from build123d import *

# Parameters (mm, degrees)
SKETCH1_W           = 88.9
SKETCH1_H           = 30.48
BOSS_EXTRUDE1_DEPTH = 3.175
BOSS_EXTRUDE2_DEPTH = 10.16
SKETCH3_W           = 68.58
SKETCH3_H           = 20.32
SKETCH3_W_2         = 10.16
CUT_EXTRUDE1_DEPTH  = 95.751277696
SKETCH5_R           = 2.8448
CUT_EXTRUDE2_DEPTH  = 12.7
CUT_EXTRUDE3_DEPTH  = 95.399536545
FILLET1_R           = 2.54


# Read off the part's stored shape, not the designer's step: Mirror4
with BuildPart() as part:
    # Sketch1 → Boss-Extrude1 (new body)
    with BuildSketch(Plane(origin=(0, 0, 0), x_dir=(1, 0, 0), z_dir=(0, 1, 0))):
        with Locations((-44.45, -15.24)):
            Rectangle(SKETCH1_W, SKETCH1_H)
    extrude(amount=BOSS_EXTRUDE1_DEPTH)

    # Sketch2 → Boss-Extrude2 (add)
    with BuildSketch(Plane.XY.offset(30.48)):
        with BuildLine():
            Line((-68.58, 3.175), (-65.151, 12.065))
            Line((-65.151, 12.065), (-54.991, 12.065))
            ThreePointArc((-54.991, 12.065), (-46.99, 4.064), (-38.989, 12.065))
            Line((-38.989, 12.065), (-28.829, 12.065))
            Line((-28.829, 12.065), (-25.4, 3.175))
            Line((-25.4, 3.175), (-68.58, 3.175))
        make_face()
    extrude(amount=-BOSS_EXTRUDE2_DEPTH)

    # Sketch3 → Cut-Extrude1 (cut, through all)
    with BuildSketch(Plane(origin=(0, 0, 0), x_dir=(1, 0, 0), z_dir=(0, 1, 0))):
        with Locations((-54.61, -10.16)):
            Rectangle(SKETCH3_W, SKETCH3_H)
        with Locations((-5.08, -10.16)):
            Rectangle(SKETCH3_W_2, SKETCH3_H)
    extrude(amount=CUT_EXTRUDE1_DEPTH, mode=Mode.SUBTRACT)

    # Sketch5 → Cut-Extrude2 (cut)
    with BuildSketch(Plane(origin=(0, 12.065, 0), x_dir=(1, 0, 0), z_dir=(0, 1, 0))):
        with Locations(Location((-33.909, -25.4, 0), (0, 0, 180))):
            Circle(SKETCH5_R)
        with Locations(Location((-60.071, -25.4, 0), (0, 0, 180))):
            Circle(SKETCH5_R)
    extrude(amount=-CUT_EXTRUDE2_DEPTH, mode=Mode.SUBTRACT)

    # Sketch6 → Cut-Extrude3 (cut, through all)
    with BuildSketch(Plane(origin=(0, 3.175, 0), x_dir=(1, 0, 0), z_dir=(0, 1, 0))):
        with BuildLine():
            Line((-81.28, -23.0505), (-73.66, -23.0505))
            ThreePointArc((-73.66, -23.0505), (-71.3105, -25.4), (-73.66, -27.7495))
            Line((-73.66, -27.7495), (-81.28, -27.7495))
            ThreePointArc((-81.28, -27.7495), (-83.6295, -25.4), (-81.28, -23.0505))
        make_face()
        with BuildLine():
            Line((-17.78, -23.0505), (-10.16, -23.0505))
            ThreePointArc((-10.16, -23.0505), (-7.8105, -25.4), (-10.16, -27.7495))
            Line((-10.16, -27.7495), (-17.78, -27.7495))
            ThreePointArc((-17.78, -27.7495), (-20.1295, -25.4), (-17.78, -23.0505))
        make_face()
    extrude(amount=-CUT_EXTRUDE3_DEPTH, mode=Mode.SUBTRACT)

    # Mirror4: part across plane


with BuildPart() as part_1:
    add(part.part)
    add(part.part.mirror(Plane.XY))

    # Fillet1
    fillet1_edges = [part_1.edges().sort_by_distance(p)[0] for p in [
        (0, 3.175, 25.4),
        (-88.9, 1.5875, -30.48),
        (0, 3.175, -25.4),
        (-78.74, 3.175, -30.48),
        (0, 1.5875, -30.48),
        (-12.7, 3.175, -30.48),
        (-68.58, 3.175, -25.4),
        (-27.1145, 7.62, -30.48),
        (-25.4, 3.175, -25.4),
        (-66.8655, 7.62, -30.48),
        (-27.1145, 7.62, -20.32),
        (-66.8655, 7.62, -20.32),
        (-12.7, 3.175, 30.48),
        (-88.9, 3.175, -25.4),
        (-22.86, 3.175, -20.32),
        (-78.74, 3.175, -20.32),
        (-88.9, 1.5875, -20.32),
        (-20.32, 1.5875, -20.32),
        (-25.4, 3.175, 25.4),
        (-66.8655, 7.62, 20.32),
        (0, 1.5875, -20.32),
        (-68.58, 3.175, 25.4),
        (-5.08, 3.175, -20.32),
        (-10.16, 1.5875, -20.32),
        (-27.1145, 7.62, 20.32),
        (-27.1145, 7.62, 30.48),
        (-66.8655, 7.62, 30.48),
        (-88.9, 3.175, 25.4),
        (-22.86, 3.175, 20.32),
        (-78.74, 3.175, 20.32),
        (-88.9, 1.5875, 20.32),
        (-20.32, 3.175, 0),
        (-20.32, 1.5875, 20.32),
        (0, 1.5875, 20.32),
        (-10.16, 3.175, 0),
        (-5.08, 3.175, 20.32),
        (-10.16, 1.5875, 20.32),
        (-78.74, 3.175, 30.48),
        (0, 1.5875, 30.48),
        (-88.9, 1.5875, 30.48),
    ]]
    fillet(fillet1_edges, radius=FILLET1_R)


solid = part_1.part
CAD build for the part. Positions are in the model's coordinates, mm. A direction names the side the tool comes from. Round coordinates to 2 decimals unless told otherwise and drop trailing zeros. Write each loop counter-clockwise with the first axis right and the second up, starting at its lowest first coordinate (ties: lowest second). Pieces come first, ordered by that corner, then holes. Notation, with made-up numbers: (-24.75, 12.25) -> (21.25, 12.25) arc R20 ccw to (21.25, 40.25) -> close; hole circle Ø9 at (-11.5, -4). An arc over 180 degrees is marked (long way). Answer as a JSON object with one key per item and string values.
(1) Band-saw the part on A-A, the plane z = 25.4. Count the separate pieces of the cut face and the enclosed holes in it, then the cut area to 3 significant figures.
Reported:
{"separate pieces": "5", "enclosed holes": "0", "area": "318 mm^2"}
(2) Which spindle directions (+Z, -Z, +X, -X, +Y, -Y) get a long thin tool onto all of the face, cutting with end or side? Do faces 4 (the face through (-5.116, 2.411, 21.044)), 5 (the face through (-78.454, 2.451, -21.084)), 6 (the face through (-48, 3, -20.32)). Say none if no direction does.
Reported:
{"face 4": "+X, +Y", "face 5": "-X, +Y", "face 6": "-X, +Y, -Y"}
(3) Band-saw the part on B-B, the plane x = -50.5. List the corners of the cut face in (y, z).
Reported:
{"outline": "(0, -30.48) -> (4.88, -30.48) -> (4.88, -20.32) -> (0, -20.32) -> close; (0, 20.32) -> (4.88, 20.32) -> (4.88, 30.48) -> (0, 30.48) -> close"}
(4) Two-plate mould, pull along X, no slides. Class faces 1 (the face through (-88.176, 2.411, -25.364)), 2 (the face through (-25.08, 3.61, -25.36)), 3 (the face through (-20.13, 1.61, 25.45)): +X half, -X half, draft (parallel to the pull), parting line (faces both ways), or undercut.
Reported:
{"face 1": "-X half", "face 2": "+X half", "face 3": "undercut"}
(5) Pin check, flat tips, straight feed: P1, Ø3, axis at y = 2.5, z = 3, coming from the +X side; P2, Ø4, axis at x = -45, z = 23.5, coming from the +Y side; P3, Ø1, axis at x = -16, y = 1.5, coming from the -Z side. Stop position of each tip, or through.
Reported:
{"P1": "stops at x = -10.19", "P2": "stops at y = 5.13", "P3": "stops at z = -30.45"}
(6) Probe probe 1 along Z at (x, y) = (-60, 4); probe 2 along X at (y, z) = (9.5, -25.4); probe 3 along X at (y, z) = (7, 27). List the from-to ranges inside material, lowest first. Write a range as [from, to].
Reported:
{"probe 1": "z = [-30.48, -28.24], [-22.56, -20.32], [20.32, 22.56], [28.24, 30.48]", "probe 2": "x = [-66.14, -62.92], [-57.23, -54.57], [-39.41, -36.75], [-31.06, -27.84]", "probe 3": "x = [-67.1, -62.42], [-57.72, -53.18], [-40.8, -36.26], [-31.56, -26.88]"}
(7) Band-saw the part on D-D, the plane z = 9.5. List the corners of the cut face in (x, y) (3 decimals).
Reported:
{"outline": "(-20.32, 0) -> (-10.16, 0) -> (-10.16, 0.635) arc R2.54 ccw to (-12.7, 3.175) -> (-17.78, 3.175) arc R2.54 ccw to (-20.32, 0.635) -> close"}
